```python
from build123d import *

# Parameters (mm, degrees)
SKETCH1_W           = 269.8
SKETCH1_H           = 142.5
BOSS_EXTRUDE2_DEPTH = 15
SKETCH2_W           = 239.8
SKETCH2_H           = 112.5
CUT_EXTRUDE1_DEPTH  = 5
BOSS_EXTRUDE3_DEPTH = 75
SKETCH7_R           = 8.089056034
SKETCH7_R_2         = 3.089056034
BOSS_EXTRUDE4_DEPTH = 15
SKETCH12_R          = 8.089056034
SKETCH12_R_2        = 3.089056034
BOSS_EXTRUDE5_DEPTH = 15
SKETCH14_W          = 17.02273013
SKETCH14_H          = 15
CUT_EXTRUDE2_DEPTH  = 5


with BuildPart() as part:
    # Sketch1 → Boss-Extrude2 (new body)
    with BuildSketch(Plane(origin=(0, 0, 0), x_dir=(1, 0, 0), z_dir=(0, 1, 0))):
        with Locations((-23.308401977, 12.292504119)):
            Rectangle(SKETCH1_W, SKETCH1_H)
    extrude(amount=BOSS_EXTRUDE2_DEPTH)

    # Sketch2 → Cut-Extrude1 (cut)
    with BuildSketch(Plane(origin=(0, 15, 0), x_dir=(1, 0, 0), z_dir=(0, 1, 0))):
        with Locations((-23.308401977, 12.292504119)):
            Rectangle(SKETCH2_W, SKETCH2_H)
    extrude(amount=-CUT_EXTRUDE1_DEPTH, mode=Mode.SUBTRACT)

    # Sketch3 → Boss-Extrude3 (add)
    with BuildSketch(Plane(origin=(0, 15, 0), x_dir=(1, 0, 0), z_dir=(0, 1, 0))):
        Polygon((-143.208401977, 68.542504119), (-158.208401977, 68.542504119), (-158.208401977, 83.542504119), (111.591598023, 83.542504119), (111.591598023, 68.542504119), align=None)
    extrude(amount=BOSS_EXTRUDE3_DEPTH)

    # Sketch7 → Boss-Extrude4 (add)
    with BuildSketch(Plane(origin=(-143.208401977, 0, 0), x_dir=(0, 0, -1), z_dir=(1, 0, 0))):
        with Locations((76.070987498, 95.45383679)):
            Circle(SKETCH7_R)
        with Locations((76.070987498, 95.45383679)):
            Circle(SKETCH7_R_2, mode=Mode.SUBTRACT)
    extrude(amount=-BOSS_EXTRUDE4_DEPTH)

    # Sketch12 → Boss-Extrude5 (add)
    with BuildSketch(Plane.ZY.offset(-96.591598023)):
        with Locations((-76.070987498, 95.45383679)):
            Circle(SKETCH12_R)
        with Locations((-76.070987498, 95.45383679)):
            Circle(SKETCH12_R_2, mode=Mode.SUBTRACT)
    extrude(amount=-BOSS_EXTRUDE5_DEPTH)

    # Sketch14 → Cut-Extrude2 (cut)
    with BuildSketch(Plane(origin=(0, 90, 0), x_dir=(1, 0, 0), z_dir=(0, 1, 0))):
        Polygon((-126.208401977, 83.542504119), (-128.208401977, 83.542504119), (-143.208401977, 83.542504119), (-143.208401977, 82.044972081), (-143.208401977, 70.097002915), (-143.208401977, 68.542504119), (-128.208401977, 68.542504119), (-126.208401977, 68.542504119), align=None)
        with Locations((88.080232958, 76.042504119)):
            Rectangle(SKETCH14_W, SKETCH14_H)
    extrude(amount=-CUT_EXTRUDE2_DEPTH, mode=Mode.SUBTRACT)


solid = part.part
```
Input: part model. Units: mm. Frame: model coordinates. A direction names the side the tool comes from. Coordinates: 2 decimals unless noted, no trailing zeros. Order: outer loops, then holes, each group sorted by start corner. A loop starts at its lowest first (then second) coordinate and runs counter-clockwise, first axis right, second up. Notation, with made-up numbers: (3, 86.25) - (45, 86.25) arc R26 cw to (45, 106.25) - close; hole circle Ø7 at (-15.5, -5.5). An arc over 180 degrees is marked (long way). Return JSON: item names as keys, results as strings.
Q1. Cut plane C-C (y = 60.5). Return loops of the section in (x, z).
The answers:
{"outline": "(-158.21, -83.54) - (111.59, -83.54) - (111.59, -68.54) - (-158.21, -68.54) - close"}
Q2. Cut plane B-B (z = -47). Return loops of the section in (x, y).
The answers:
{"outline": "(-158.21, 0) - (111.59, 0) - (111.59, 15) - (96.59, 15) - (96.59, 10) - (-143.21, 10) - (-143.21, 15) - (-158.21, 15) - close"}
Q3. Draft query along Z for faces 4 (the flat face through (-25, 44, -83.543)), 5 (the flat face through (-25, 10, -13)), 6 (the flat face through (-126.208, 88, -76)). Return one class per face: +Z half, -Z half, draft (parallel to the pull), parting line (faces both ways), or undercut.
The answers:
{"face 4": "-Z half", "face 5": "undercut", "face 6": "draft"}
Q4. Cut plane A-A (x = 50.5). Return loops of the section in (y, z), then the cut area to 3 significant figures.
The answers:
{"outline": "(0, -83.54) - (90, -83.54) - (90, -68.54) - (10, -68.54) - (10, 43.96) - (15, 43.96) - (15, 58.96) - (0, 58.96) - close", "area": "2,700 mm2"}
Q5. Ray query, probe 1 along X at (y, z) = (11, -28); probe 2 along Y at (x, z) = (61, -54); probe 3 along Z at (x, y) = (2.5, 47). Return the intervals inside material, ascending.
The answers:
{"probe 1": "x = -158.21 to -143.21, 96.59 to 111.59", "probe 2": "y = 0 to 10", "probe 3": "z = -83.54 to -68.54"}
Q6. First-contact query: pin 1 (1 mm diameter, centred on x = -9.5, z = 23, fed in from +Y); pin 2 (1.2 mm diameter, centred on x = -153, z = -69.5, fed in from +Y); pin 3 (1.5 mm diameter, centred on x = -10, y = 12.5, fed in from -Z). Flat tips, straight axial feed; report the tip coordinate or a pass-through.
The answers:
{"pin 1": "stops at y = 10", "pin 2": "stops at y = 100.91", "pin 3": "stops at z = -83.54"}
Q7. Access query for faces 1 (the flat face through (111.592, 14, -39)), 2 (the flat face through (-143.208, 13, -12)), 3 (the flat face through (79.569, 88, -76)). Directions: +Z, -Z, +X, -X, +Y, -Y. A direction counts if a zero-diameter tool reaches every point of the face in a straight line with its end or side. Return the directions, or none.
The answers:
{"face 1": "+Z, -Z, +X, +Y, -Y", "face 2": "+Y", "face 3": "+Z, -Z, +Y"}
